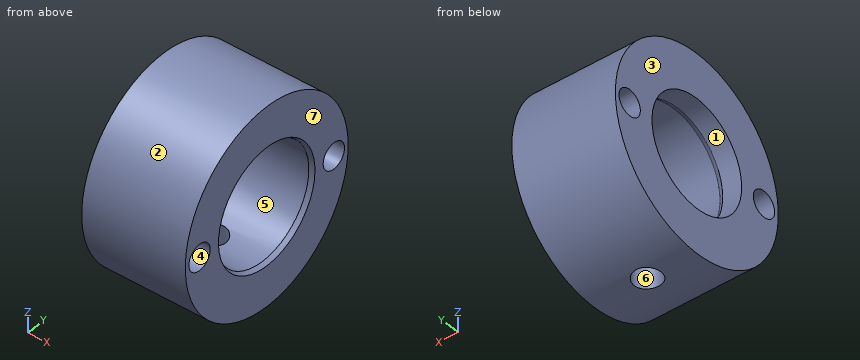
```python
from build123d import *

# Parameters (mm, degrees)
F0_R     = 31.75
F0_R_2   = 4.1656
F1_DEPTH = 33.3248
F4_R     = 4.3053
F5_DEPTH = 32.512


with BuildPart() as f1:
    # F0 (on Right) → F1 (new body)
    with BuildSketch(Plane.YZ):
        Circle(F0_R)
        with Locations((-26.1874, 0)):
            Circle(F0_R_2, mode=Mode.SUBTRACT)
        with Locations((26.1874, 0)):
            Circle(F0_R_2, mode=Mode.SUBTRACT)
    extrude(amount=-F1_DEPTH)

    # F2 (on Front) → F3 (revolve, cut)
    with BuildSketch(Plane.XZ):
        Polygon((0, 18.811576), (-1.4224, 18.1483), (-25.8064, 18.1483), (-27.222632, 17.4879), (-34.925, 17.4879), (-34.925, 0), (0, 0), align=None)
    revolve(axis=Axis((-17.4625, 0, 0), (1, 0, 0)), mode=Mode.SUBTRACT)

    # F4 (on Top) → F5 (cut)
    with BuildSketch(Plane.XY):
        with Locations((-17.4752, 0)):
            Circle(F4_R)
    extrude(amount=-F5_DEPTH, mode=Mode.SUBTRACT)


solid = f1.part
```
Design review of the part built by this model. Coordinates are the model's own, in mm. Face numbers are marked on the shaded views. A direction names the side the tool comes from. Give positions to 0.01 mm unless a question says otherwise; leave off trailing zeros. Write each loop counter-clockwise with the first axis right and the second up, starting at its lowest first coordinate (ties: lowest second). Pieces come first, ordered by that corner, then holes. Notation, with made-up numbers: (19, 3.5) - (60, 3.5) arc R19 ccw to (60, 22.5) - close; hole circle Ø11 at (78.25, 55). An arc over 180 degrees is marked (long way). Return JSON: item names as keys, results as strings. Group by question number.
(1) Insertion check: pin 1 (10 mm diameter, centred on x = -10, z = 18, fed in from +Y); pin 2 (4 mm diameter, centred on x = -11.5, y = 5.5, fed in from -Z); pin 3 (11 mm diameter, centred on x = -17.48, y = 0, fed in from +Z); pin 4 (7.5 mm diameter, centred on y = -26.19, z = 0, fed in from -X). Each pin has a flat end and moves straight along its axis. Give the tip position at first contact, or say it passes through.
(2) We need section B-B, the plane z = 0. Give the boundary of the cut face in (x, y).
(3) We need section C-C, the plane x = -5.5. Give the boundary of the cut face in (y, z).
(4) We need section A-A, the plane y = 0. Give the boundary of the cut face in (x, z), then the cut area to 3 significant figures.
(5) Mouldability with a two-part tool opening along Y and no side actions: class the marked faces 1, 2, 3 and 4 as +Y half, -Y half, draft (parallel to the pull), parting line (faces both ways), or undercut.
(6) To check wall thickness, follow probe 1 along Y at (x, z) = (-18, 2); probe 2 along Z at (x, y) = (-29.5, 0.5); probe 3 along X at (y, z) = (0, -23.5). State the ranges of each line that lie inside material, in increasing order.
(7) We need section D-D, the plane z = -23.5. Give the boundary of the cut face in (x, y).
(8) Machinability: for the marked faces 5, 6 and 7, which of the approach directions +Z, -Z, +X, -X, +Y, -Y give a long, thin tool a straight path to every point of the face, cutting with its end or side? Answer none if there is none.
Reported:
{
 "1": {"pin 1": "stops at y = 28.97", "pin 2": "stops at z = -31.56", "pin 3": "stops at z = 31.75", "pin 4": "passes through"},
 "2": {"outline": "(-33.32, -31.75) - (0, -31.75) - (0, -30.35) - (-33.32, -30.35) - close; (-33.32, -22.02) - (0, -22.02) - (0, -18.81) - (-1.42, -18.15) - (-25.81, -18.15) - (-27.22, -17.49) - (-33.32, -17.49) - close; (-33.32, 17.49) - (-27.22, 17.49) - (-25.81, 18.15) - (-1.42, 18.15) - (0, 18.81) - (0, 22.02) - (-33.32, 22.02) - close; (-33.32, 30.35) - (0, 30.35) - (0, 31.75) - (-33.32, 31.75) - close"},
 "3": {"outline": "circle Ø63.5 at (0, 0); hole circle Ø8.33 at (-26.19, 0); hole circle Ø36.3 at (0, 0); hole circle Ø8.33 at (26.19, 0)"},
 "4": {"outline": "(-33.32, -31.75) - (-21.78, -31.75) - (-21.78, -18.15) - (-25.81, -18.15) - (-27.22, -17.49) - (-33.32, -17.49) - close; (-33.32, 17.49) - (-27.22, 17.49) - (-25.81, 18.15) - (-1.42, 18.15) - (0, 18.81) - (0, 31.75) - (-33.32, 31.75) - close; (-13.17, -31.75) - (0, -31.75) - (0, -18.81) - (-1.42, -18.15) - (-13.17, -18.15) - close", "area": "797 mm2"},
 "5": {"face 1": "undercut", "face 2": "parting line", "face 3": "draft", "face 4": "undercut"},
 "6": {"probe 1": "y = -31.69 to -29.84, -22.53 to -18.04, 18.04 to 22.53, 29.84 to 31.69", "probe 2": "z = -31.75 to -17.48, 17.48 to 31.75", "probe 3": "x = -33.32 to -21.78, -13.17 to 0"},
 "7": {"outline": "(-33.32, -21.35) - (0, -21.35) - (0, 21.35) - (-33.32, 21.35) - close; hole circle Ø8.61 at (-17.48, 0)"},
 "8": {"face 5": "+X", "face 6": "-Z", "face 7": "+Z, -Z, +X, +Y, -Y"}
}
